Design review of the part shown in the three views and the two pictorial views. Dimensions are in mm from the part's minimum x, y and z. A direction names the side the tool comes from. Coordinates: 2 decimals unless noted, no trailing zeros. Write each loop counter-clockwise with the first axis right and the second up, starting at its lowest first coordinate (ties: lowest second). Pieces come first, ordered by that corner, then holes.
Q1. For L1, parallel to Z at x = 31, y = 9.5; L2, parallel to Y at x = 52.5, z = 14; L3, parallel to X at y = 8.75, z = 38, list the stretches that pass through material, from the lowest coordinate up.
Q2. Take a section at B-B, the plane z = 36. Write out the cut boundary in (x, y).
Q3. For pin 1 Ø1.5 at (y, z) = (8, 9.5) entering from -X; pin 2 Ø5 at (x, y) = (44.5, 3) entering from -Z, all flat-tipped, find the tip position at first contact; note any pin that passes through.
Q4. For the marked faces 4 and 5, list the 3-axis set-ups (+Z, -Z, +X, -X, +Y, -Y) from which the entire face can be reached by the end or side of a thin tool; tool diameter is ignored.
Q5. Take a section at D-D, the plane x = 54. Write out the cut boundary in (y, z).
Q6. Take a section at A-A, the plane x = 31. Write out the cut boundary in (y, z), plus the area to 3 significant figures.
Q7. The part is to be moulded in two halves that separate along X. For the marked faces 1, 2 and 3, say which applies: released by +X, released by -X, zero draft, split by the parting line, or undercut.
Q8. Take a section at C-C, the plane y = 10.5. Write out the cut boundary in (x, z).
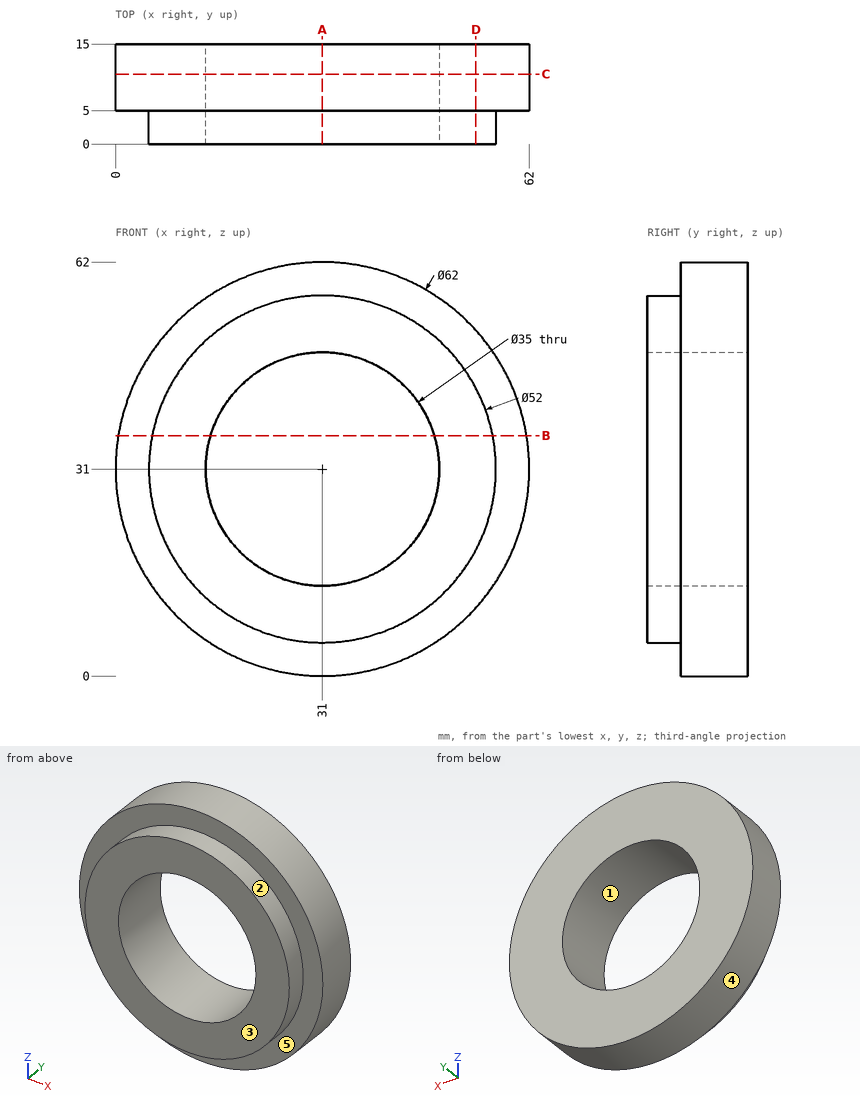
Responses:
1. L1: z = 0 to 13.5, 48.5 to 62
1. L2: y = 5 to 15
1. L3: x = 0.8 to 14.96, 47.04 to 61.2
2. outline: (0.41, 5) - (5.49, 5) - (5.49, 0) - (14.23, 0) - (14.23, 15) - (0.41, 15) - close; (47.77, 0) - (56.51, 0) - (56.51, 5) - (61.59, 5) - (61.59, 15) - (47.77, 15) - close
3. pin 1: stops at x = 7.97
3. pin 2: stops at z = 2.42
4. face 4: +Y, -Y
4. face 5: -Y
5. outline: (0, 18.88) - (5, 18.88) - (5, 10.22) - (15, 10.22) - (15, 51.78) - (5, 51.78) - (5, 43.12) - (0, 43.12) - close
6. outline: (0, 5) - (5, 5) - (5, 0) - (15, 0) - (15, 13.5) - (0, 13.5) - close; (0, 48.5) - (15, 48.5) - (15, 62) - (5, 62) - (5, 57) - (0, 57) - close
6. area: 355 mm2
7. face 1: undercut
7. face 2: split by the parting line
7. face 3: zero draft
8. outline: circle Ø62 at (31, 31); hole circle Ø35 at (31, 31)
